Input: part model. Units: mm. Frame: model coordinates. Face numbers are marked on the shaded views. A direction names the side the tool comes from. Coordinates: 2 decimals unless noted, no trailing zeros. Order: outer loops, then holes, each group sorted by start corner. A loop starts at its lowest first (then second) coordinate and runs counter-clockwise, first axis right, second up. Notation, with made-up numbers: M -36.75,24.5 L -3.75,24.5 A24 ccw -3.75,44.5 Z; hole C 9.25,53.25 d10. An arc over 180 degrees is marked long. One line per item, written item: value.
```python
from build123d import *

# Parameters (mm, degrees)
F0_R     = 12.7
F1_DEPTH = 19.05
F2_R     = 15.2691244528
F2_R_2   = 12.7
F3_DEPTH = 2.54
F4_R     = 12.475880284
F5_DEPTH = 5.08
F6_R     = 3.81


with BuildPart() as f1:
    # F0 (on Top) → F1 (new body)
    with BuildSketch(Plane.XY):
        Circle(F0_R)
    extrude(amount=F1_DEPTH)

    # F2 (on face) → F3 (join)
    with BuildSketch(Plane.XY.offset(19.05)):
        Circle(F2_R)
        Circle(F2_R_2, mode=Mode.SUBTRACT)
        Circle(F2_R_2)
    extrude(amount=F3_DEPTH)

    # F4 (on face) → F5 (join)
    with BuildSketch(Plane.XY.offset(21.59)):
        Circle(F4_R)
    extrude(amount=F5_DEPTH)

    # F6
    f6_edges = [f1.edges().sort_by_distance(p)[0] for p in [
        (-12.47588, 0, 26.67),
    ]]
    fillet(f6_edges, radius=F6_R)


solid = f1.part
```
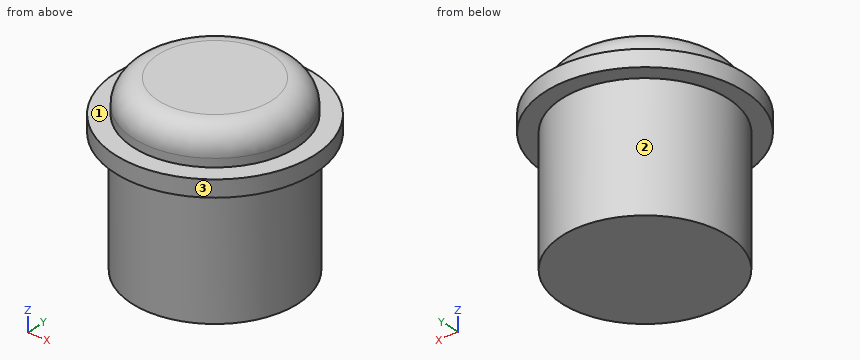
(1) Access query for the marked faces 1, 2 and 3. Directions: +Z, -Z, +X, -X, +Y, -Y. A direction counts if a zero-diameter tool reaches every point of the face in a straight line with its end or side. Return the directions, or none.
Data:
face 1: +Z
face 2: -Z
face 3: +Z, -Z
(2) First-contact query: pin 1 (12 mm diameter, centred on y = 4, z = 8.5, fed in from +X); pin 2 (3 mm diameter, centred on x = -11, z = 8, fed in from +Y); pin 3 (12 mm diameter, centred on x = -6.5, z = 11.5, fed in from -Y). Flat tips, straight axial feed; report the tip coordinate or a pass-through.
Data:
pin 1: stops at x = 12.7
pin 2: stops at y = 8.43
pin 3: stops at y = -12.69
(3) Cut plane C-C on z = 7.75. Output: boundary loops of the cut face in (x, y).
Data:
outline: C 0,0 d25.4
(4) Ray query, line 1 (Y direction, x = -0.5, z = 15.5); line 2 (Z direction, x = 13, y = 6); line 3 (Z direction, x = 7, y = 10.5). Return the intervals inside material, ascending. Write a range as from..to.
Data:
line 1: y = -12.69..12.69
line 2: z = 19.05..21.59
line 3: z = 0..21.59
(5) Cut plane A-A on x = 0. Output: boundary loops of the cut face in (y, z).
Data:
outline: M -15.27,19.05 L -12.7,19.05 L -12.7,0 L 12.7,0 L 12.7,19.05 L 15.27,19.05 L 15.27,21.59 L 12.48,21.59 L 12.48,22.86 A3.81 ccw 8.67,26.67 L -8.67,26.67 A3.81 ccw -12.48,22.86 L -12.48,21.59 L -15.27,21.59 Z
(6) Cut plane D-D on z = 20. Output: boundary loops of the cut face in (x, y).
Data:
outline: C 0,0 d30.54
